from build123d import *

# Parameters (mm, degrees)
EXTRUDE_1_DEPTH          = 125
EXTRUDE_1_DEPTH_BACK     = 125
SKETCH_1_W               = 9
SKETCH_1_H               = 6.5
CUT_EXTRUDE_1_DEPTH      = 125
CUT_EXTRUDE_1_DEPTH_BACK = 125
SKETCH_2_W               = 0.95
SKETCH_2_H               = 1.48
CHAMFER_2_SIZE           = 0.5
SKETCH_3_R               = 3
CUT_EXTRUDE_2_DEPTH      = 3.5
SKETCH_4_R               = 1.75
CUT_EXTRUDE_3_DEPTH      = 5


with BuildPart() as part:
    # 草图1 → 凸台-拉伸1 (new, two sides: drawn at the far end of the back side and taken through both)
    with BuildSketch(Plane(origin=(0, 0, 0), x_dir=(1, 0, 0), z_dir=(0, 1, 0)).offset(-EXTRUDE_1_DEPTH_BACK)):
        Rectangle(SKETCH_1_W, SKETCH_1_H)
    extrude(amount=EXTRUDE_1_DEPTH + EXTRUDE_1_DEPTH_BACK)

    # 草图2 → 切除-拉伸1 (cut, two sides: drawn at the far end of the back side and taken through both)
    with BuildSketch(Plane(origin=(0, 0, 0), x_dir=(1, 0, 0), z_dir=(0, 1, 0)).offset(-CUT_EXTRUDE_1_DEPTH_BACK)):
        with Locations((4.025, 1.15)):
            Rectangle(SKETCH_2_W, SKETCH_2_H)
        with Locations((-4.025, 1.15)):
            Rectangle(SKETCH_2_W, SKETCH_2_H)
    extrude(amount=CUT_EXTRUDE_1_DEPTH + CUT_EXTRUDE_1_DEPTH_BACK, mode=Mode.SUBTRACT)

    # 倒角2
    chamfer_2_edges = [part.edges().sort_by_distance(p)[0] for p in [
        (4.5, 0, 3.25),
        (-4.5, 0, 3.25),
        (-4.5, 0, -3.25),
        (4.5, 0, -3.25),
    ]]
    chamfer(chamfer_2_edges, length=CHAMFER_2_SIZE)

    # 草图3 → 切除-拉伸2 (cut)
    with BuildSketch(Plane(origin=(0, 0, -3.25), x_dir=(-1, 0, 0), z_dir=(0, 0, -1))):
        with Locations((0, -120)):
            Circle(SKETCH_3_R)
        with Locations((0, -100)):
            Circle(SKETCH_3_R)
        with Locations((0, -80)):
            Circle(SKETCH_3_R)
        with Locations((0, -60)):
            Circle(SKETCH_3_R)
        with Locations((0, -40)):
            Circle(SKETCH_3_R)
        with Locations((0, -20)):
            Circle(SKETCH_3_R)
        Circle(SKETCH_3_R)
        with Locations((0, 20)):
            Circle(SKETCH_3_R)
        with Locations((0, 40)):
            Circle(SKETCH_3_R)
        with Locations((0, 60)):
            Circle(SKETCH_3_R)
        with Locations((0, 80)):
            Circle(SKETCH_3_R)
        with Locations((0, 100)):
            Circle(SKETCH_3_R)
        with Locations((0, 120)):
            Circle(SKETCH_3_R)
    extrude(amount=-CUT_EXTRUDE_2_DEPTH, mode=Mode.SUBTRACT)

    # 草图4 → 切除-拉伸3 (cut)
    with BuildSketch(Plane(origin=(0, 0, 0.25), x_dir=(-1, 0, 0), z_dir=(0, 0, -1))):
        with Locations((0, -120)):
            Circle(SKETCH_4_R)
        with Locations((0, -100)):
            Circle(SKETCH_4_R)
        with Locations((0, -80)):
            Circle(SKETCH_4_R)
        with Locations((0, -60)):
            Circle(SKETCH_4_R)
        with Locations((0, -40)):
            Circle(SKETCH_4_R)
        with Locations((0, -20)):
            Circle(SKETCH_4_R)
        Circle(SKETCH_4_R)
        with Locations((0, 20)):
            Circle(SKETCH_4_R)
        with Locations((0, 40)):
            Circle(SKETCH_4_R)
        with Locations((0, 60)):
            Circle(SKETCH_4_R)
        with Locations((0, 80)):
            Circle(SKETCH_4_R)
        with Locations((0, 100)):
            Circle(SKETCH_4_R)
        with Locations((0, 120)):
            Circle(SKETCH_4_R)
        with Locations((0, 140)):
            Circle(SKETCH_4_R)
        with Locations((0, 160)):
            Circle(SKETCH_4_R)
    extrude(amount=-CUT_EXTRUDE_3_DEPTH, mode=Mode.SUBTRACT)


solid = part.part
For this review, take the finished solid that the model builds, in its own axes (mm). Round coordinates to 2 decimals unless told otherwise and drop trailing zeros. Loops run counter-clockwise (first coordinate to the right, second up) from the corner with the lowest first, then second, coordinate; pieces in that order, holes last. Notation, with made-up numbers: (84.25, 76) - (88.25, 76) arc R18 cw to (88.25, 107) - close; hole circle Ø3 at (-32, 3.25). An arc over 180 degrees is marked (long way). One line per question, with ' | ' between items.
Q1. Take a section at B-B (y = 47). Give the boundary of the cut face in (x, z).
Taken from the geometry:
outline: (-4.5, -2.75) - (-4, -3.25) - (4, -3.25) - (4.5, -2.75) - (4.5, -1.89) - (3.55, -1.89) - (3.55, -0.41) - (4.5, -0.41) - (4.5, 2.75) - (4, 3.25) - (-4, 3.25) - (-4.5, 2.75) - (-4.5, -0.41) - (-3.55, -0.41) - (-3.55, -1.89) - (-4.5, -1.89) - close
Q2. For pin 1 (2 mm diameter, centred on x = 0, y = 80, fed in from -Z); pin 2 (3 mm diameter, centred on x = 0.5, y = 21, fed in from -Z), all flat-tipped, find the tip position at first contact; note any pin that passes through.
Taken from the geometry:
pin 1: passes through | pin 2: stops at z = 0.25
Q3. The part is to be moulded in two halves that separate along X. For faces 1 (the flat face through (0, -125, 0)), 2 (the flat face through (0, -22, 0.25)), say which applies: released by +X, released by -X, zero draft, split by the parting line, or undercut.
Taken from the geometry:
face 1: zero draft | face 2: undercut
Q4. For line 1 along X through (y, z) = (100, 1.3); line 2 along Z through (x, y) = (3.75, -30.5); line 3 along Z through (x, y) = (2.25, -101), list the stretches that pass through material, from the lowest coordinate up. Write a range as [from, to].
Taken from the geometry:
line 1: x = [-4.5, -1.75], [1.75, 4.5] | line 2: z = [-3.25, -1.89], [-0.41, 3.25] | line 3: z = [0.25, 3.25]
Q5. Take a section at A-A (z = 1.25). State how many separate pieces and enclosed holes the cut face has, and give its area (3 significant figures).
Taken from the geometry:
separate pieces: 1 | enclosed holes: 13 | area: 2,120 mm²
